Could you check a few things on this model? Use its own coordinates, in mm. Give positions to 0.01 mm unless a question says otherwise; leave off trailing zeros. Write each loop counter-clockwise with the first axis right and the second up, starting at its lowest first coordinate (ties: lowest second). Pieces come first, ordered by that corner, then holes. Notation, with made-up numbers: (13, -28) - (37, -28) arc R23 ccw to (37, -11) - close; hole circle Ø10 at (-33.5, 9.5). An arc over 180 degrees is marked (long way). Answer as a JSON object with one key per item and string values. Group by question number.
Solid Edge part; units mm, degrees
sketch "Sketch1" plane through (0, 0, 0) normal (0, 0, 1) x (1, 0, 0)
  circle A0 centre (-133.4653, -62.7673) radius 2.9988
  circle A1 centre (-133.4653, -162.7673) radius 2.9988
  circle A2 centre (60.674, 131.0545) radius 2.9988
  circle A3 centre (160.674, 131.0545) radius 2.9988
  line L0 (-118.1099, -234.2368) -> (-153.4653, -198.8815)
  line L1 (-153.4653, -198.8815) -> (-153.4653, -24.9332)
  line L2 (24.0185, 152.5506) -> (-153.4653, -24.9332)
  line L3 (197.9668, 152.5506) -> (24.0185, 152.5506)
  line L4 (197.9668, 152.5506) -> (233.3222, 117.1952)
  line L5 (233.3222, 117.1952) -> (-118.1099, -234.2368)
  dimension "D1" = 233.3222
  dimension "D2" = 197.9668
  dimension "D3" = 133.4653
  dimension "D4" = 60.674
  dimension "D5" = 60.674
  dimension "D6" = 197.9668
extrude "Protrusion1" add sketch "Sketch1" along normal blind 3
properties material "Nylon, allgemein"
(1) I want a section at C-C, the plane x = 88.5. Please give me the cut outline in (y, z).
(2) I want a section at B-B, the plane y = -207.5. Please give me the cut outline in (x, z).
(3) I need wall thicknesses on L1, parallel to Y at x = -133, z = 2.2; L2, parallel to X at y = -164, z = 1.3; L3, parallel to X at y = -182, z = 1.75. Which ranges of each line are inside material? Lowest first, please.
(4) I want a section at A-A, the plane z = 1.9. Please give me the cut outline in (x, y), and give its area (3 significant figures).
(5) Will this pin go through, and if not, where does the flat tip stop? P1, Ø1.5, axis at x = -1.5, z = 2.5, coming from the -Y side.
Entries:
{
 "1": {"outline": "(-27.63, 0) - (152.55, 0) - (152.55, 3) - (-27.63, 3) - close"},
 "2": {"outline": "(-144.85, 0) - (-91.37, 0) - (-91.37, 3) - (-144.85, 3) - close"},
 "3": {"L1": "-219.35 to -165.73, -159.8 to -65.73, -59.8 to -4.47", "L2": "-153.47 to -136.2, -130.73 to -47.87", "L3": "-153.47 to -65.87"},
 "4": {"outline": "(-153.47, -198.88) - (-118.11, -234.24) - (233.32, 117.2) - (197.97, 152.55) - (24.02, 152.55) - (-153.47, -24.93) - close; hole circle Ø6 at (-133.47, -162.77); hole circle Ø6 at (-133.47, -62.77); hole circle Ø6 at (60.67, 131.05); hole circle Ø6 at (160.67, 131.05)", "area": "70,700 mm^2"},
 "5": {"P1": "y = -118.38"}
}
